Input: part model. Units: mm. Frame: model coordinates. Face numbers are marked on the shaded views. Coordinates: 2 decimals unless noted, no trailing zeros. Order: outer loops, then holes, each group sorted by start corner. A loop starts at its lowest first (then second) coordinate and runs counter-clockwise, first axis right, second up. Notation, with made-up numbers: (-26.75, 67) - (9.25, 67) arc R26 ccw to (9.25, 89) - close; hole circle Ø5 at (6, 0). An arc over 180 degrees is marked (long way). One line per question, with ' | ' between items.
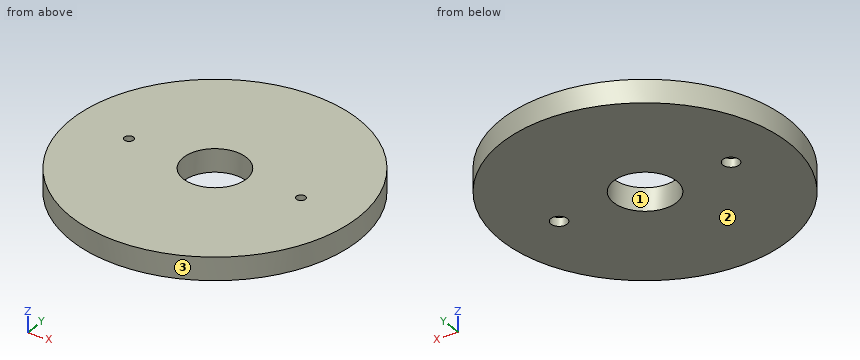
from build123d import *

# Parameters (mm, degrees)
ESQUISSE1_R             = 50
ESQUISSE1_R_2           = 11
BOSS_EXTRU_1_DEPTH      = 8
ESQUISSE2_R             = 1.6
ENL_V_MAT_EXTRU_1_DEPTH = 72.161787499
ESQUISSE3_R             = 2.85
ENL_V_MAT_EXTRU_2_DEPTH = 3


with BuildPart() as part:
    # Esquisse1 → Boss.-Extru.1 (new body)
    with BuildSketch(Plane.XY):
        Circle(ESQUISSE1_R)
        Circle(ESQUISSE1_R_2, mode=Mode.SUBTRACT)
    extrude(amount=BOSS_EXTRU_1_DEPTH)

    # Esquisse2 → Enlèv. mat.-Extru.1 (cut, through all)
    with BuildSketch(Plane(origin=(0, 0, 0), x_dir=(-1, 0, 0), z_dir=(0, 0, -1))):
        with Locations((30, 0)):
            Circle(ESQUISSE2_R)
        with Locations((-30, 0)):
            Circle(ESQUISSE2_R)
    extrude(amount=-ENL_V_MAT_EXTRU_1_DEPTH, mode=Mode.SUBTRACT)

    # Esquisse3 → Enlèv. mat.-Extru.2 (cut)
    with BuildSketch(Plane(origin=(0, 0, 0), x_dir=(-1, 0, 0), z_dir=(0, 0, -1))):
        with Locations((30, 0)):
            Circle(ESQUISSE3_R)
        with Locations((-30, 0)):
            Circle(ESQUISSE3_R)
    extrude(amount=-ENL_V_MAT_EXTRU_2_DEPTH, mode=Mode.SUBTRACT)


solid = part.part
Item 1: Section B-B on y = 0. Return the cut outline in (x, z).
Data:
outline: (-50, 0) - (-32.85, 0) - (-32.85, 3) - (-31.6, 3) - (-31.6, 8) - (-50, 8) - close; (-28.4, 3) - (-27.15, 3) - (-27.15, 0) - (-11, 0) - (-11, 8) - (-28.4, 8) - close; (11, 0) - (27.15, 0) - (27.15, 3) - (28.4, 3) - (28.4, 8) - (11, 8) - close; (31.6, 3) - (32.85, 3) - (32.85, 0) - (50, 0) - (50, 8) - (31.6, 8) - close
Item 2: Contact query for flat-ended pins moving along their axis: P1, Ø9, axis at x = 30, y = 0, coming from the +Z side; P2, Ø3, axis at x = -16, z = 6.5, coming from the -Y side; P3, Ø4.5, axis at x = -30, y = 0, coming from the -Z side; P4, Ø1, axis at x = 7, z = 1, coming from the -Y side. Output: stop coordinate, or through.
Data:
P1: z = 8 | P2: y = -47.85 | P3: z = 3 | P4: y = -49.58
Item 3: Section A-A on x = -30. Return the cut outline in (y, z).
Data:
outline: (-40, 0) - (-2.85, 0) - (-2.85, 3) - (-1.6, 3) - (-1.6, 8) - (-40, 8) - close; (1.6, 3) - (2.85, 3) - (2.85, 0) - (40, 0) - (40, 8) - (1.6, 8) - close
Item 4: Draft query along X for the marked faces 1, 2 and 3. Return one class per face: released by +X, released by -X, zero draft, split by the parting line, or undercut.
Data:
face 1: undercut | face 2: zero draft | face 3: split by the parting line
Item 5: Section D-D on x = 0. Return the cut outline in (y, z).
Data:
outline: (-50, 0) - (-11, 0) - (-11, 8) - (-50, 8) - close; (11, 0) - (50, 0) - (50, 8) - (11, 8) - close
Item 6: Ray query, line 1 (Y direction, x = 0, z = 5.25); line 2 (X direction, y = 10, z = 7); line 3 (Y direction, x = 30, z = 1.9). Return the intervals inside material, ascending.
Data:
line 1: -50 to -11, 11 to 50 | line 2: -48.99 to -4.58, 4.58 to 48.99 | line 3: -40 to -2.85, 2.85 to 40
Item 7: Section C-C on z = 1.5. Return the cut outline in (x, y), and give its area (3 significant figures).
Data:
outline: circle Ø100 at (0, 0); hole circle Ø5.7 at (-30, 0); hole circle Ø22 at (0, 0); hole circle Ø5.7 at (30, 0) | area: 7,420 mm^2
